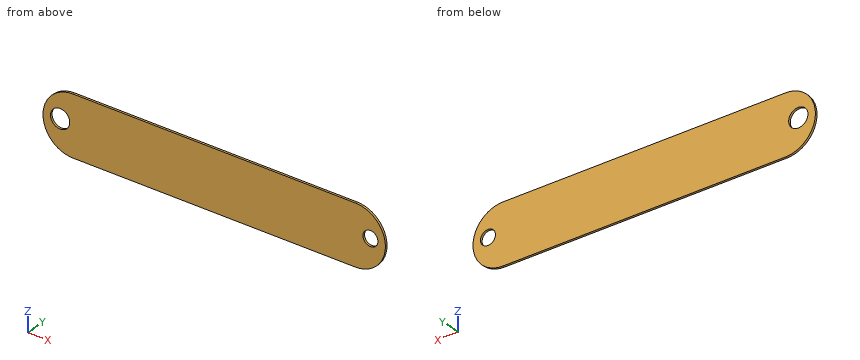
```python
from build123d import *

# Parameters (mm, degrees)
SKETCH_1_W      = 80
SKETCH_1_H      = 14
SKETCH_1_R      = 2.25
SKETCH_1_R_2    = 1.75
EXTRUDE_1_DEPTH = 0.5
FILLET_1_R      = 7


with BuildPart() as part:
    # 草图1 → 凸台-拉伸1 (new body)
    with BuildSketch(Plane(origin=(0, 0, 0), x_dir=(1, 0, 0), z_dir=(0, 1, 0))):
        with Locations((40, -7)):
            Rectangle(SKETCH_1_W, SKETCH_1_H)
        with Locations(Location((4, -7.5, 0), (0, 0, 270))):
            Circle(SKETCH_1_R, mode=Mode.SUBTRACT)
        with Locations(Location((76.5, -7.5, 0), (0, 0, 270))):
            Circle(SKETCH_1_R_2, mode=Mode.SUBTRACT)
    extrude(amount=EXTRUDE_1_DEPTH)

    # 圆角1
    fillet_1_edges = [part.edges().sort_by_distance(p)[0] for p in [
        (0, 0.25, 0),
        (80, 0.25, 0),
        (80, 0.25, 14),
        (0, 0.25, 14),
    ]]
    fillet(fillet_1_edges, radius=FILLET_1_R - 0.0001)  # a hair under: the kernel refuses the full size


solid = part.part
```
CAD build for the part. Positions are in the model's coordinates, mm. Coordinates: 2 decimals unless noted, no trailing zeros. Loops run counter-clockwise (first coordinate to the right, second up) from the corner with the lowest first, then second, coordinate; pieces in that order, holes last. Notation, with made-up numbers: (15, -17.5) - (62, -17.5) arc R20 ccw to (62, -5.5) - close; hole circle Ø1 at (37, 13). An arc over 180 degrees is marked (long way). Return JSON: item names as keys, results as strings.
1. Band-saw the part on C-C (x = 4). Give the cut face in (y, z), and give its area (3 significant figures).
Result:
{"outline": "(0, 0.68) - (0.5, 0.68) - (0.5, 5.25) - (0, 5.25) - close; (0, 9.75) - (0.5, 9.75) - (0.5, 13.32) - (0, 13.32) - close", "area": "4.07 mm2"}
2. Band-saw the part on A-A (x = 76.5). Give the cut face in (y, z).
Result:
{"outline": "(0, 0.94) - (0.5, 0.94) - (0.5, 5.75) - (0, 5.75) - close; (0, 9.25) - (0.5, 9.25) - (0.5, 13.06) - (0, 13.06) - close"}
3. Probe L1, parallel to X at y = 0.4, z = 7.5; L2, parallel to Z at x = 76.5, y = 0.2; L3, parallel to X at y = 0.4, z = 9.5. List the from-to ranges inside material, lowest first. Write a range as from..to.
Result:
{"L1": "x = 0.02..1.75, 6.25..74.75, 78.25..79.98", "L2": "z = 0.94..5.75, 9.25..13.06", "L3": "x = 0.46..2.97, 5.03..79.54"}
4. Band-saw the part on B-B (y = 0.1). State how many separate pieces and enclosed holes the cut face has, and give its area (3 significant figures).
Result:
{"separate pieces": "1", "enclosed holes": "2", "area": "1,050 mm2"}
5. Band-saw the part on D-D (z = 1). Give the cut face in (x, y).
Result:
{"outline": "(3.39, 0) - (76.61, 0) - (76.61, 0.5) - (3.39, 0.5) - close"}
6. Drop a flat-ended pin along its axis: pin 1 (6 mm diameter, centred on x = 64, z = 7.5, fed in from -Y). Give the stop position or say it passes through.
Result:
{"pin 1": "stops at y = 0"}
